CAD build for the part. Positions are in the model's coordinates, mm. Face numbers are marked on the shaded views. A direction names the side the tool comes from. Coordinates: 2 decimals unless noted, no trailing zeros. Order: outer loops, then holes, each group sorted by start corner. A loop starts at its lowest first (then second) coordinate and runs counter-clockwise, first axis right, second up. Notation, with made-up numbers: (88.5, 13) - (110.5, 13) arc R30 ccw to (110.5, 35) - close; hole circle Ø11 at (11.25, -29.5). An arc over 180 degrees is marked (long way). Use one line per item in the form item = value.
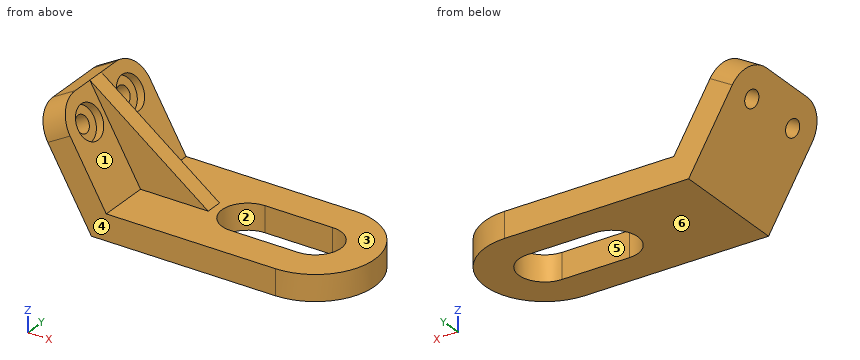
```python
from build123d import *

# Parameters (mm, degrees)
F1_DEPTH  = 44.704
F3_DEPTH  = 9.652
F4_DEPTH  = 9.652
F8_DEPTH  = 3.175
F9_R      = 3.175
F10_DEPTH = 9.652
F9_R_2    = 6.35
F11_DEPTH = 3.175
F12_R     = 10.922


with BuildPart() as f1:
    # F0 (on Front) → F1 (new body)
    with BuildSketch(Plane.XZ):
        Polygon((-21.8362923991, 37.8215678842), (0, 0), (69.0725847982, 0), (69.0725847982, 9.652), (5.5725847982, 9.652), (-13.4774152018, 42.6475678842), align=None)
    extrude(amount=-F1_DEPTH)

    # F2 (on face) → F3 (join, through all)
    with BuildSketch(Plane.XY.offset(9.652)):
        with BuildLine():
            Line((69.0725847982, 12.7), (69.0725847982, 0))
            ThreePointArc((69.0725847982, 0), (91.4245847982, 22.352), (69.0725847982, 44.704))
            Line((69.0725847982, 44.704), (69.0725847982, 32.004))
            ThreePointArc((69.0725847982, 32.004), (78.7245847982, 22.352), (69.0725847982, 12.7))
        make_face()
    extrude(amount=-F3_DEPTH)

    # F2 (on face) → F4 (cut, through all)
    with BuildSketch(Plane.XY.offset(9.652)):
        with BuildLine():
            Line((43.6725847982, 12.7), (69.0725847982, 12.7))
            Line((69.0725847982, 12.7), (69.0725847982, 32.004))
            Line((69.0725847982, 32.004), (43.6725847982, 32.004))
            ThreePointArc((43.6725847982, 32.004), (34.0205847982, 22.352), (43.6725847982, 12.7))
        make_face()
    extrude(amount=-F4_DEPTH, mode=Mode.SUBTRACT)

    # F7 (on offset) → F8 (join, symmetric)
    with BuildSketch(Plane.XZ.offset(-22.352)):
        Polygon((30.9725847982, 9.652), (-13.4774152018, 42.6475678842), (5.5725847982, 9.652), align=None)
    extrude(amount=F8_DEPTH, both=True)

    # F9 (on face) → F10 (cut, through all)
    with BuildSketch(Plane(origin=(8.3588771973, 0, 4.826), x_dir=(0, 1, 0), z_dir=(0.8660254038, 0, 0.5))):
        with Locations((10.922, 32.7505847982)):
            Circle(F9_R)
        with BuildLine():
            ThreePointArc((30.607, 32.7505847982), (33.782, 29.5755847982), (36.957, 32.7505847982))
            Line((36.957, 32.7505847982), (33.782, 32.7505847982))
            Line((33.782, 32.7505847982), (30.607, 32.7505847982))
        make_face()
        with BuildLine():
            Line((33.782, 32.7505847982), (36.957, 32.7505847982))
            ThreePointArc((36.957, 32.7505847982), (33.782, 35.9255847982), (30.607, 32.7505847982))
            Line((30.607, 32.7505847982), (33.782, 32.7505847982))
        make_face()
    extrude(amount=-F10_DEPTH, mode=Mode.SUBTRACT)

    # F9 (on face) → F11 (cut)
    with BuildSketch(Plane(origin=(8.3588771973, 0, 4.826), x_dir=(0, 1, 0), z_dir=(0.8660254038, 0, 0.5))):
        with Locations((10.922, 32.7505847982)):
            Circle(F9_R_2)
        with Locations((10.922, 32.7505847982)):
            Circle(F9_R, mode=Mode.SUBTRACT)
        with BuildLine():
            ThreePointArc((27.432, 32.7505847982), (33.782, 26.4005847982), (40.132, 32.7505847982))
            Line((40.132, 32.7505847982), (36.957, 32.7505847982))
            ThreePointArc((36.957, 32.7505847982), (33.782, 29.5755847982), (30.607, 32.7505847982))
            Line((30.607, 32.7505847982), (27.432, 32.7505847982))
        make_face()
        with BuildLine():
            Line((36.957, 32.7505847982), (40.132, 32.7505847982))
            ThreePointArc((40.132, 32.7505847982), (33.782, 39.1005847982), (27.432, 32.7505847982))
            Line((27.432, 32.7505847982), (30.607, 32.7505847982))
            ThreePointArc((30.607, 32.7505847982), (33.782, 35.9255847982), (36.957, 32.7505847982))
        make_face()
    extrude(amount=-F11_DEPTH, mode=Mode.SUBTRACT)

    # F12
    f12_edges = [f1.edges().sort_by_distance(p)[0] for p in [
        (-17.656854, 0, 40.234568),
        (-17.656854, 44.704, 40.234568),
    ]]
    fillet(f12_edges, radius=F12_R)


solid = f1.part
```
Item 1: 3-axis set-ups, long thin cutter, end or side, ignore diameter. For the marked faces 1, 2 and 3: which of +Z, -Z, +X, -X, +Y, -Y reach the whole face in a straight line?
Derived:
face_1 = +Z, +X, -Y
face_2 = +Z, -Z
face_3 = +Z, +X
Item 2: Cut at B-B, the plane y = 9.5. Write the cut outline in (x, z).
Derived:
outline = (-21.79, 37.74) - (-17.79, 30.82) - (-12.19, 34.06) - (-13.86, 36.96) - (-11.11, 38.55) - (-13.43, 42.57) - close; (-14.96, 25.9) - (0, 0) - (87.36, 0) - (87.36, 9.65) - (5.57, 9.65) - (-4.92, 27.83) - (-7.67, 26.24) - (-9.35, 29.14) - close
Item 3: Drop flat-ended pins along their axis: pin 1 (12 mm diameter, centred on y = 10.5, z = 31, fed in from -X); pin 2 (4 mm diameter, centred on x = -10, y = 22.5, fed in from -Z). Give the stop position or say it passes through.
Derived:
pin_1 = -21.36
pin_2 = 13.86
Item 4: Cut at C-C, the plane z = 17.5. Write the cut outline in (x, y).
Derived:
outline = (-10.1, 0) - (1.04, 0) - (1.04, 19.18) - (20.4, 19.18) - (20.4, 25.53) - (1.04, 25.53) - (1.04, 44.7) - (-10.1, 44.7) - close
Item 5: Cut at A-A, the plane x = 59. Write the cut outline in (y, z).
Derived:
outline = (0, 0) - (12.7, 0) - (12.7, 9.65) - (0, 9.65) - close; (32, 0) - (44.7, 0) - (44.7, 9.65) - (32, 9.65) - close
Item 6: Two-plate mould, pull along Y, no slides. Class the marked faces 4, 5 and 6: +Y half, -Y half, draft (parallel to the pull), parting line (faces both ways), or undercut.
Derived:
face_4 = -Y half
face_5 = undercut
face_6 = draft
Item 7: Cut at D-D, the plane x = 29. Write the cut outline in (y, z), plus the area to 3 significant figures.
Derived:
outline = (0, 0) - (44.7, 0) - (44.7, 9.65) - (25.53, 9.65) - (25.53, 11.12) - (19.18, 11.12) - (19.18, 9.65) - (0, 9.65) - close
area = 441 mm²
Item 8: Drill centre lines: line 1 (Z direction, x = 30, y = 37.5); line 2 (X direction, y = 17, z = 8.5); line 3 (X direction, y = 37, z = 30). Where is each one in solid material? Low to high. Write a range as [from, to].
Derived:
line_1 = [0, 9.65]
line_2 = [-4.91, 35.64], [77.1, 90.77]
line_3 = [-17.32, -9.84]
